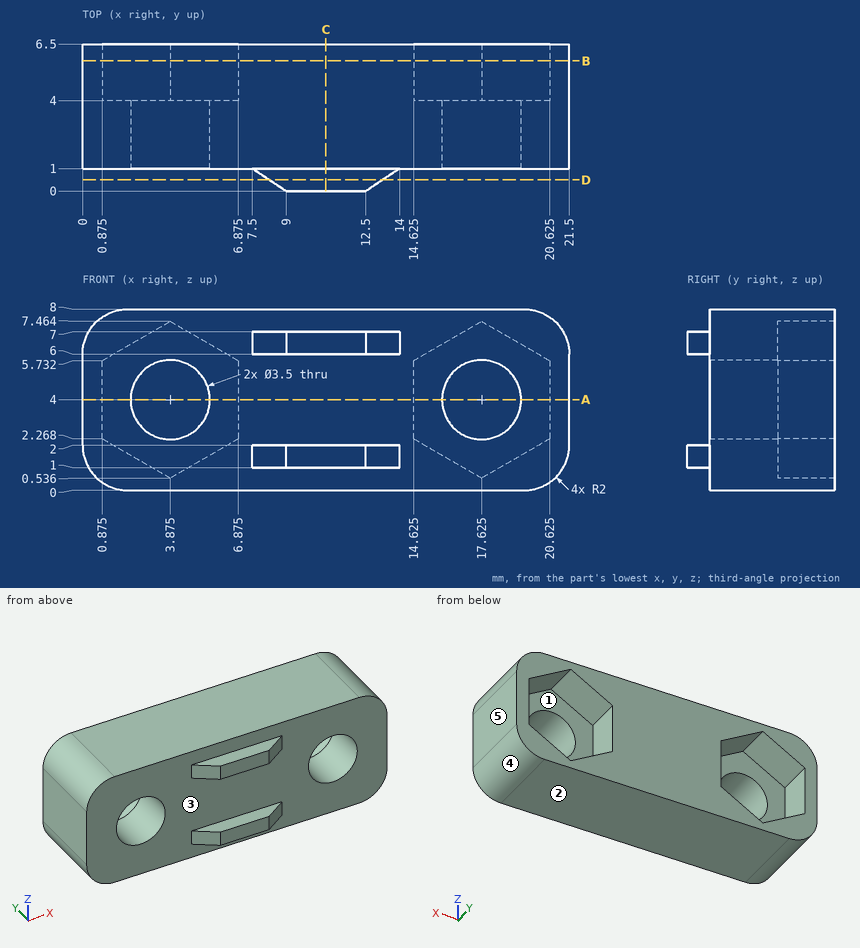
For this review, use the dimensioned drawing (mm, ordinates from the lowest corner) and the shaded views. A direction names the side the tool comes from. Give positions to 0.01 mm unless a question says otherwise; leave off trailing zeros. Order: outer loops, then holes, each group sorted by start corner. A loop starts at its lowest first (then second) coordinate and runs counter-clockwise, first axis right, second up. Notation, with made-up numbers: M -39.75,34 L -16.75,34 A24 ccw -16.75,46 Z; hole C 73.25,72 d6. An arc over 180 degrees is marked long. One line per question, with ' | ' between items. Start each with the question number.
1) Clearance check with flat-ended pins moving along their axes: P1, Ø3, axis at x = 17.625, z = 4, coming from the +Y side; P2, Ø1, axis at x = 10, z = 4.5, coming from the -Y side; P3, Ø0.8, axis at x = 10, y = 0.5, coming from the +Z side; P4, Ø0.5, axis at x = 11.5, y = 0.5, coming from the -Z side. State where each tip first meets the part, or that it passes through.
2) Consider section D-D, the plane y = 0.5. Give the boundary of the cut face in (x, z).
3) Consider section B-B, the plane y = 5.75. Give the boundary of the cut face in (x, z) (3 decimals).
4) Mouldability with a two-part tool opening along Z and no side actions: class the marked faces 3, 4 and 5 as pulls with the +Z half, pulls with the -Z half, needs draft (parallel to the pull), parting line crosses it, or undercut.
5) For the marked faces 1 and 2, list the 3-axis set-ups (+Z, -Z, +X, -X, +Y, -Y) from which the entire face can be reached by the end or side of a thin tool; tool diameter is ignored.
6) Consider section C-C, the plane x = 10.75. Give the boundary of the cut face in (y, z), then the cut area to 3 significant figures.
7) Wall thickness on L1, parallel to X at y = 5.25, z = 4 (3 decimals); L2, parallel to Y at x = 13, z = 3.5; L3, parallel to X at y = 2.75, z = 5: over which ranges is each line inside the solid? List them lowest first. Write a range as from..to.
8) Consider section A-A, the plane z = 4. Give the boundary of the cut face in (x, y) (3 decimals).
Found:
1) P1: passes through | P2: stops at y = 1 | P3: stops at z = 7 | P4: stops at z = 1
2) outline: M 8.25,1 L 13.25,1 L 13.25,2 L 8.25,2 Z; M 8.25,6 L 13.25,6 L 13.25,7 L 8.25,7 Z
3) outline: M 0,2 A2 ccw 2,0 L 19.5,0 A2 ccw 21.5,2 L 21.5,6 A2 ccw 19.5,8 L 2,8 A2 ccw 0,6 Z; hole M 0.875,2.268 L 3.875,0.536 L 6.875,2.268 L 6.875,5.732 L 3.875,7.464 L 0.875,5.732 Z; hole M 14.625,2.268 L 17.625,0.536 L 20.625,2.268 L 20.625,5.732 L 17.625,7.464 L 14.625,5.732 Z
4) face 3: undercut | face 4: pulls with the -Z half | face 5: needs draft
5) face 1: +Y | face 2: -Z, +X, -X, +Y, -Y
6) outline: M 0,1 L 1,1 L 1,0 L 6.5,0 L 6.5,8 L 1,8 L 1,7 L 0,7 L 0,6 L 1,6 L 1,2 L 0,2 Z | area: 46.0 mm²
7) L1: x = 0..0.875, 6.875..14.625, 20.625..21.5 | L2: y = 1..6.5 | L3: x = 0..2.44, 5.31..16.19, 19.06..21.5
8) outline: M 0,1 L 2.125,1 L 2.125,4 L 0.875,4 L 0.875,6.5 L 0,6.5 Z; M 5.625,1 L 15.875,1 L 15.875,4 L 14.625,4 L 14.625,6.5 L 6.875,6.5 L 6.875,4 L 5.625,4 Z; M 19.375,1 L 21.5,1 L 21.5,6.5 L 20.625,6.5 L 20.625,4 L 19.375,4 Z
